Check sheet for the modelled part. Datum: model origin and axes. Units: mm. A direction names the side the tool comes from. Round coordinates to 2 decimals unless told otherwise and drop trailing zeros. Write each loop counter-clockwise with the first axis right and the second up, starting at its lowest first coordinate (ties: lowest second). Pieces come first, ordered by that corner, then holes.
Item 1: Material ranges on line 1 along Z through (x, y) = (0, 19); line 2 along Z through (x, y) = (0, 35.5); line 3 along Z through (x, y) = (0, 21), recorded low to high.
Item 2: Depth check by flat-ended pin: pin 1 (12 mm diameter, centred on x = 8.5, y = 19, fed in from +Z); pin 2 (1.3 mm diameter, centred on x = -7.5, y = 18.5, fed in from +Z); pin 3 (6 mm diameter, centred on x = -9, z = 3, fed in from +Y). Enter the tip coordinate at first touch or a pass-through.
Item 3: Section check C-C, the plane z = -5. Record the cut outline in (x, y).
Item 4: Release check for a two-part mould opening along Y. For faces 1 (the flat face through (0, 1.588, 0)), 2 (the flat face through (15.438, 22, -10)), 3 (the flat face through (-0.2, 0.5, -20.9)), 4 (the flat face through (0, 25, -15.844)) record: pulls with the +Y half, pulls with the -Y half, needs draft (parallel to the pull), parting line crosses it, or undercut.
Item 5: Set-up check for faces 5 (the flat face through (0, 31.75, -18)), 6 (the flat face through (-14.93, 10.29, -20.91)), 7 (the cylindrical face through (13.21, 22.72, -4.16)): record each of +Z, -Z, +X, -X, +Y, -Y from which the full face is reachable in a straight line by a thin tool's end or side.
Item 6: Section check B-B, the plane x = 0. Record the cut outline in (y, z), plus the area to 3 significant figures.
from build123d import *

# Parameters (mm, degrees)
SKETCH1_R           = 13.85
BOSS_EXTRUDE1_DEPTH = 44.45
SKETCH2_R           = 15.08125
BOSS_EXTRUDE2_DEPTH = 1.5875
CUT_EXTRUDE1_DEPTH  = 31.875
CHAMFER1_SIZE       = 1


with BuildPart() as part:
    # Sketch1 → Boss-Extrude1 (new body)
    with BuildSketch(Plane(origin=(0, 0, 0), x_dir=(1, 0, 0), z_dir=(0, 1, 0))):
        with BuildLine():
            Line((-15.4375, 0), (-15.4375, 21.4))
            Line((-15.4375, 21.4), (15.4375, 21.4))
            Line((15.4375, 21.4), (15.4375, 0))
            ThreePointArc((15.4375, 0), (0, -15.4375), (-15.4375, 0))
        make_face()
        Circle(SKETCH1_R, mode=Mode.SUBTRACT)
    extrude(amount=BOSS_EXTRUDE1_DEPTH)

    # Sketch2 → Boss-Extrude2 (add)
    with BuildSketch(Plane.XZ):
        Circle(SKETCH2_R)
    extrude(amount=-BOSS_EXTRUDE2_DEPTH)

    # Sketch3 → Cut-Extrude1 (cut, through all)
    with BuildSketch(Plane(origin=(15.4375, 0, 0), x_dir=(0, 0, -1), z_dir=(1, 0, 0))):
        Polygon((21.4, 30.1625), (19.8125, 30.1625), (19.8125, 31.75), (15.84375, 31.75), (15.84375, 18.25625), (19.8125, 18.25625), (19.8125, 19.84375), (21.4, 19.84375), align=None)
    extrude(amount=-CUT_EXTRUDE1_DEPTH, mode=Mode.SUBTRACT)

    # Chamfer1
    chamfer1_edges = [part.edges().sort_by_distance(p)[0] for p in [
        (0, 44.45, -21.4),
        (-15.4375, 44.45, -10.7),
        (-15.4375, 9.921875, -21.4),
        (15.4375, 9.921875, -21.4),
        (0, 44.45, 15.4375),
        (-15.4375, 0, -10.7),
        (0, 0, -21.4),
        (15.4375, 0, -10.7),
        (0, 0, 15.4375),
        (15.4375, 44.45, -10.7),
        (-15.4375, 37.30625, -21.4),
        (15.4375, 37.30625, -21.4),
    ]]
    chamfer(chamfer1_edges, length=CHAMFER1_SIZE)


solid = part.part
Values found:
1. line 1: z = -21.4 to -19.81, -15.84 to -13.85, 13.85 to 15.44
1. line 2: z = -21.4 to -13.85, 13.85 to 15.44
1. line 3: z = -15.84 to -13.85, 13.85 to 15.44
2. pin 1: stops at z = 15.23
2. pin 2: stops at z = 13.83
2. pin 3: stops at y = 1.59
3. outline: (-15.44, 1) - (-14.44, 0) - (14.44, 0) - (15.44, 1) - (15.44, 43.45) - (14.44, 44.45) - (12.92, 44.45) - (12.92, 1.59) - (-12.92, 1.59) - (-12.92, 44.45) - (-14.44, 44.45) - (-15.44, 43.45) - close
4. face 1: pulls with the +Y half
4. face 2: needs draft
4. face 3: pulls with the -Y half
4. face 4: undercut
5. face 5: +X, -X
5. face 6: -Z, -X, +Y, -Y
5. face 7: +Y
6. outline: (0, -20.4) - (1, -21.4) - (19.84, -21.4) - (19.84, -19.81) - (18.26, -19.81) - (18.26, -15.84) - (31.75, -15.84) - (31.75, -19.81) - (30.16, -19.81) - (30.16, -21.4) - (43.45, -21.4) - (44.45, -20.4) - (44.45, -13.85) - (1.59, -13.85) - (1.59, 13.85) - (44.45, 13.85) - (44.45, 14.44) - (43.45, 15.44) - (1, 15.44) - (0, 14.44) - close
6. area: 378 mm2
